```python
from build123d import *

# Parameters (mm, degrees)
SKETCH1_W           = 41
SKETCH1_H           = 41
BOSS_EXTRUDE1_DEPTH = 41
CHAMFER1_SIZE       = 5
SKETCH2_R           = 5
CUT_EXTRUDE1_DEPTH  = 42


with BuildPart() as part:
    # Sketch1 → Boss-Extrude1 (new body)
    with BuildSketch(Plane(origin=(0, 0, 0), x_dir=(1, 0, 0), z_dir=(0, 1, 0))):
        Rectangle(SKETCH1_W, SKETCH1_H)
    extrude(amount=BOSS_EXTRUDE1_DEPTH)

    # Chamfer1
    chamfer1_edges = [part.edges().sort_by_distance(p)[0] for p in [
        (20.5, 20.5, 20.5),
        (-20.5, 20.5, 20.5),
        (-20.5, 20.5, -20.5),
        (20.5, 20.5, -20.5),
    ]]
    chamfer(chamfer1_edges, length=CHAMFER1_SIZE)

    # Sketch2 → Cut-Extrude1 (cut, through all)
    with BuildSketch(Plane.XZ):
        Circle(SKETCH2_R)
    extrude(amount=-CUT_EXTRUDE1_DEPTH, mode=Mode.SUBTRACT)


solid = part.part
```
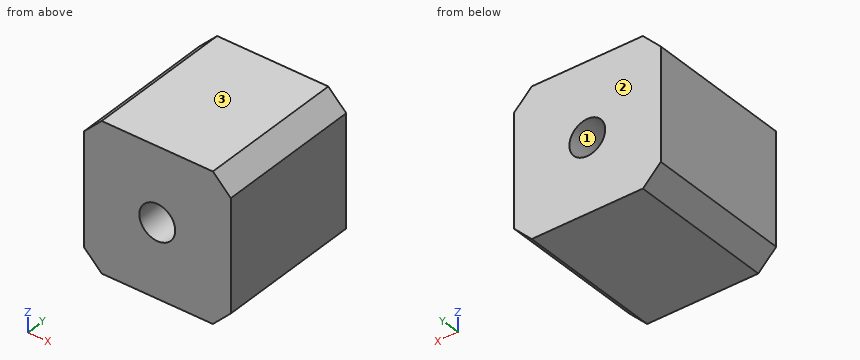
Read the model definition and answer for the solid it produces. Units are mm, in the model's axes. Face numbers are marked on the shaded views. Give positions to 0.01 mm unless a question says otherwise; leave off trailing zeros. Write each loop counter-clockwise with the first axis right and the second up, starting at its lowest first coordinate (ties: lowest second). Pieces come first, ordered by that corner, then holes. Notation, with made-up numbers: (14, 35.5) -> (73, 35.5) arc R21 cw to (73, 70.5) -> close; hole circle Ø9 at (18, 81). An arc over 180 degrees is marked (long way). Answer as a JSON object with one key per item and string values.
1) Section A-A on z = 0 is taken. Write down the section's boundary in (x, y).
Findings below:
{"outline": "(-20.5, 0) -> (-5, 0) -> (-5, 41) -> (-20.5, 41) -> close; (5, 0) -> (20.5, 0) -> (20.5, 41) -> (5, 41) -> close"}
2) Section C-C on x = 18.5 is taken. Write down the section's boundary in (y, z).
Findings below:
{"outline": "(0, -17.5) -> (41, -17.5) -> (41, 17.5) -> (0, 17.5) -> close"}
3) Straight lines are drawn through the part: probe 1 along Z at (x, y) = (0, 17); probe 2 along Z at (x, y) = (-17.5, 4.5); probe 3 along X at (y, z) = (7, 18.5). For each, find the intervals that lie inside material, in ascending order. Write a range as from..to.
Findings below:
{"probe 1": "z = -20.5..-5, 5..20.5", "probe 2": "z = -18.5..18.5", "probe 3": "x = -17.5..17.5"}
4) For a pull along Z with two mould halves and no side action, classify the marked faces 1, 2 and 3 as pulls with the +Z half, pulls with the -Z half, needs draft (parallel to the pull), parting line crosses it, or undercut.
Findings below:
{"face 1": "undercut", "face 2": "needs draft", "face 3": "pulls with the +Z half"}
5) Section B-B on x = 0 is taken. Write down the section's boundary in (y, z), then the cut area to 3 significant figures.
Findings below:
{"outline": "(0, -20.5) -> (41, -20.5) -> (41, -5) -> (0, -5) -> close; (0, 5) -> (41, 5) -> (41, 20.5) -> (0, 20.5) -> close", "area": "1,270 mm^2"}
